Can you work these out from the model? Positions are in its coordinate system, mm. A direction names the side the tool comes from. Give positions to 0.01 mm unless a question says otherwise; leave off trailing zeros. Order: outer loops, then holes, each group sorted by start corner. A loop starts at its lowest first (then second) coordinate and runs counter-clockwise, first axis right, second up. Notation, with made-up numbers: M -30,52.5 L 21,52.5 A20 ccw 21,77.5 Z; hole C 30,53.5 d9. An arc over 180 degrees is marked long. Answer as a JSON object with one key per item and string values.
```python
from build123d import *
from build123d.topology import SkipClean

# Parameters (mm, degrees)
SKETCH1_R               = 38.1
BOSS_EXTRUDE1_DEPTH     = 76.2
SHELL2_T                = 3.175
SKETCH2_W               = 3
SKETCH2_H               = 82.55
SKETCH2_W_2             = 82.55
SKETCH2_H_2             = 3
BOSS_EXTRUDE2_DEPTH     = 7
CUT_EXTRUDE1_DEPTH      = 99.527366122
CUT_EXTRUDE1_DEPTH_BACK = 99.527366122
SKETCH3_R               = 61.906276858
SKETCH3_R_2             = 41.275
SKETCH4_R               = 20.64
CUT_EXTRUDE2_DEPTH      = 7
SCALE1_SCALE            = 0.615384615


with BuildPart() as part:
    # Sketch1 → Boss-Extrude1 (new body)
    with BuildSketch(Plane(origin=(0, 0, 0), x_dir=(1, 0, 0), z_dir=(0, 1, 0))):
        with Locations(Location((0, 0, 0), (0, 0, 90))):
            Circle(SKETCH1_R)
    extrude(amount=BOSS_EXTRUDE1_DEPTH)

    # Shell2
    shell2_openings = [part.faces().sort_by_distance(p)[0] for p in [
        (0, 76.2, 0),
    ]]
    offset(amount=SHELL2_T, openings=shell2_openings, kind=Kind.INTERSECTION)

    # Sketch2 → Boss-Extrude2 (add)
    with BuildSketch(Plane(origin=(0, -3.175, 0), x_dir=(-1, 0, 0), z_dir=(0, -1, 0))):
        Rectangle(SKETCH2_W, SKETCH2_H)
        Polygon((-23.047310797, -34.273854321), (25.47436178, 32.510498564), (23.047310797, 34.273854321), (-25.47436178, -32.510498564), align=None)
        Polygon((-38.791332219, -14.181261217), (39.718383202, 11.328091668), (38.791332219, 14.181261217), (-39.718383202, -11.328091668), align=None)
        Polygon((-39.718383202, 11.328091668), (38.791332219, -14.181261217), (39.718383202, -11.328091668), (-38.791332219, 14.181261217), align=None)
        Polygon((-25.47436178, 32.510498564), (23.047310797, -34.273854321), (25.47436178, -32.510498564), (-23.047310797, 34.273854321), align=None)
        Polygon((-14.181261217, 38.791332219), (11.328091668, -39.718383202), (14.181261217, -38.791332219), (-11.328091668, 39.718383202), align=None)
        Polygon((11.328091668, 39.718383202), (-14.181261217, -38.791332219), (-11.328091668, -39.718383202), (14.181261217, 38.791332219), align=None)
        Polygon((32.510498564, 25.47436178), (-34.273854321, -23.047310797), (-32.510498564, -25.47436178), (34.273854321, 23.047310797), align=None)
        Rectangle(SKETCH2_W_2, SKETCH2_H_2)
        Polygon((-34.273854321, 23.047310797), (32.510498564, -25.47436178), (34.273854321, -23.047310797), (-32.510498564, 25.47436178), align=None)
    extrude(amount=BOSS_EXTRUDE2_DEPTH)

    # Sketch3 → Cut-Extrude1 (cut, two sides: drawn at the far end of the back side and taken through both)
    with SkipClean():  # the faces are left unmerged after this step: merging them gives an invalid solid
        with BuildSketch(Plane.XZ.offset(3.175).offset(-CUT_EXTRUDE1_DEPTH_BACK)):
            Circle(SKETCH3_R)
            with Locations(Location((0, 0, 0), (0, 0, 272.082679548))):
                Circle(SKETCH3_R_2, mode=Mode.SUBTRACT)
        extrude(amount=CUT_EXTRUDE1_DEPTH + CUT_EXTRUDE1_DEPTH_BACK, mode=Mode.SUBTRACT)

    # Sketch4 → Cut-Extrude2 (cut)
    with SkipClean():  # the faces are left unmerged after this step: merging them gives an invalid solid
        with BuildSketch(Plane.XZ.offset(10.175)):
            Circle(SKETCH4_R)
        extrude(amount=-CUT_EXTRUDE2_DEPTH, mode=Mode.SUBTRACT)


with BuildPart() as part_1:
    # Scale1: scaled about (0, 25.742888467, 0)
    add(part.part.scale(SCALE1_SCALE).moved(Location((0, 9.901110949, 0))))


solid = part_1.part
```
1) Thinking about a two-plate mould opening in X: for faces 1 (the face through (18.464, 5.824, -5.029)), 2 (the face through (11, 3.64, -15)), 3 (the face through (-12.076, 5.763, 3.937)), which applies, pulls with the +X half, pulls with the -X half, needs draft (parallel to the pull), parting line crosses it, or undercut?
Results found:
{"face 1": "pulls with the +X half", "face 2": "needs draft", "face 3": "undercut"}
2) For faces 4 (the face through (-18.295, 5.824, -4.974)), 5 (the face through (17.894, 5.824, 6.785)), 6 (the face through (19, 6, 0.923)), 7 (the face through (18.295, 5.824, 4.974)), which set-ups out of +Z, -Z, +X, -X, +Y, -Y let a thin tool reach every point of the face, with its end or its side?
Results found:
{"face 4": "-X, -Y", "face 5": "-Y", "face 6": "+X, -X, -Y", "face 7": "+X, -Y"}
3) I'm going to push flat-ended pins straight in: pin 1 Ø4.5 at (y, z) = (6, -17) entering from +X; pin 2 Ø4 at (x, y) = (-5, 23.5) entering from +Z; pin 3 Ø4.5 at (y, z) = (6, 19) entering from -X. Where does each tip first touch, or does it pass through?
Results found:
{"pin 1": "stops at x = 20.68", "pin 2": "stops at z = 25.22", "pin 3": "stops at x = -18.05"}
4) I want a section at A-A on y = 18. Write out the boundary of the cut face in (x, z).
Results found:
{"outline": "C 0,0 d50.8; hole C 0,0 d46.89"}
5) I need wall thicknesses on L1, parallel to X at y = 38, z = 0; L2, parallel to X at y = 43.5, z = -10.5; L3, parallel to Y at x = 1, z = -6.5. Which ranges of each line are inside material? Lowest first, please.
Results found:
{"L1": "x = -25.4 to -23.45, 23.45 to 25.4", "L2": "x = -23.13 to -20.96, 20.96 to 23.13", "L3": "y = 7.95 to 9.9"}
